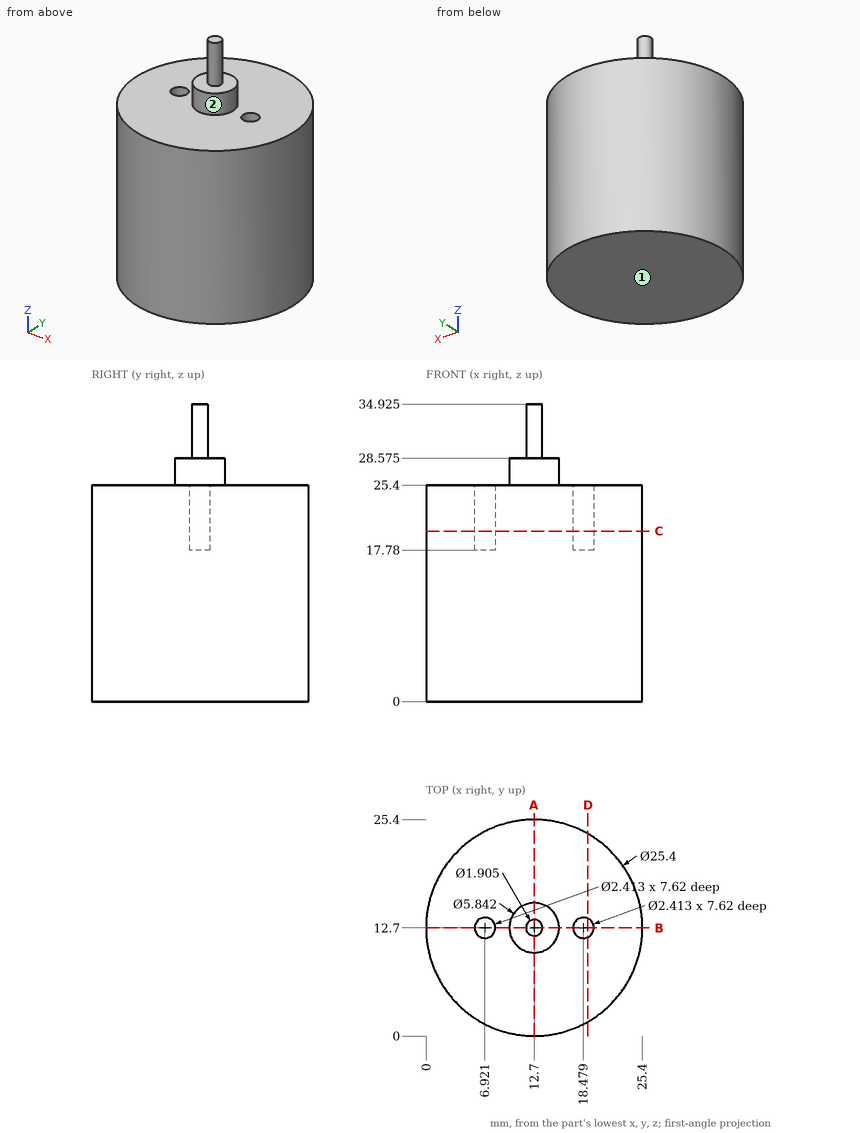
For this review, use the dimensioned drawing (mm, ordinates from the lowest corner) and the shaded views. A direction names the side the tool comes from. Round coordinates to 2 decimals unless told otherwise and drop trailing zeros. Order: outer loops, then holes, each group sorted by start corner. A loop starts at its lowest first (then second) coordinate and runs counter-clockwise, first axis right, second up. Notation, with made-up numbers: (18.25, -2.75) -> (67.25, -2.75) arc R29 cw to (67.25, 35.25) -> close; hole circle Ø6 at (65, 88). An arc over 180 degrees is marked (long way). Put each result on its own line as item: value.
Q1. Add section B-B on y = 12.7. Write out the cut boundary in (x, z) (1 decimal), plus the area to 3 significant figures.
Check result:
outline: (0, 0) -> (25.4, 0) -> (25.4, 25.4) -> (19.7, 25.4) -> (19.7, 17.8) -> (17.3, 17.8) -> (17.3, 25.4) -> (15.6, 25.4) -> (15.6, 28.6) -> (13.7, 28.6) -> (13.7, 34.9) -> (11.7, 34.9) -> (11.7, 28.6) -> (9.8, 28.6) -> (9.8, 25.4) -> (8.1, 25.4) -> (8.1, 17.8) -> (5.7, 17.8) -> (5.7, 25.4) -> (0, 25.4) -> close
area: 639 mm2
Q2. Machinability: for the marked faces 1 and 2, which of the approach directions +Z, -Z, +X, -X, +Y, -Y give a long, thin tool a straight path to every point of the face, cutting with its end or side? Answer none if there is none.
Check result:
face 1: -Z, +X, -X, +Y, -Y
face 2: +Z
Q3. Add section D-D on x = 19. Write out the cut boundary in (y, z).
Check result:
outline: (1.67, 0) -> (23.73, 0) -> (23.73, 25.4) -> (13.79, 25.4) -> (13.79, 17.78) -> (11.61, 17.78) -> (11.61, 25.4) -> (1.67, 25.4) -> close
Q4. Add section C-C on z = 20. Write out the cut boundary in (x, y) (1 decimal).
Check result:
outline: circle Ø25.4 at (12.7, 12.7); hole circle Ø2.4 at (6.9, 12.7); hole circle Ø2.4 at (18.5, 12.7)
Q5. Insertion check: pin 1 Ø1.9 at (x, y) = (18, 13) entering from +Z; pin 2 Ø10 at (x, z) = (3.5, 26.5) entering from +Y; pin 3 Ø0.7 at (x, y) = (7, 12) entering from +Z. Each pin has a flat end and moves straight along its axis. Give the tip position at first contact, or say it passes through.
Check result:
pin 1: z = 25.4
pin 2: y = 24.64
pin 3: z = 17.78
Q6. Add section A-A on x = 12.7. Write out the cut boundary in (y, z) (1 decimal), plus the area to 3 significant figures.
Check result:
outline: (0, 0) -> (25.4, 0) -> (25.4, 25.4) -> (15.6, 25.4) -> (15.6, 28.6) -> (13.7, 28.6) -> (13.7, 34.9) -> (11.7, 34.9) -> (11.7, 28.6) -> (9.8, 28.6) -> (9.8, 25.4) -> (0, 25.4) -> close
area: 676 mm2
Q7. For probe 1 along Z at (x, y) = (2.75, 17.5); probe 2 along Z at (x, y) = (15, 13.25) (1 decimal), list the stretches that pass through material, from the lowest coordinate up. Write a range as [from, to].
Check result:
probe 1: [0, 25.4]
probe 2: [0, 28.6]
